For this review, use the dimensioned drawing (mm, ordinates from the lowest corner) and the shaded views. A direction names the side the tool comes from. Give positions to 0.01 mm unless a question says otherwise; leave off trailing zeros. Write each loop counter-clockwise with the first axis right and the second up, starting at its lowest first coordinate (ties: lowest second). Pieces come first, ordered by that corner, then holes. Notation, with made-up numbers: M -23,-1.5 L -4,-1.5 A8 cw -4,13.5 Z; hole C -13.5,-6.5 d1. An arc over 180 degrees is marked long. Write each question's results on one line, items separated by ' | '. Start each with the question number.
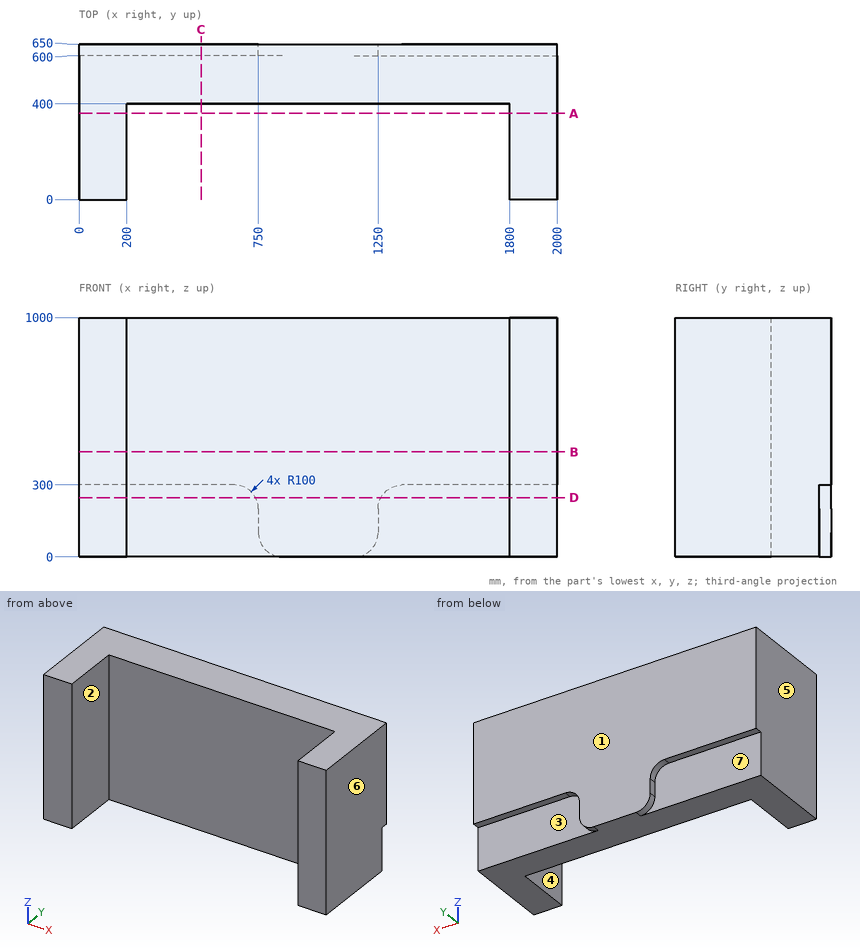
(1) Wall thickness on L1, parallel to X at y = 142, z = 559; L2, parallel to Y at x = 331, z = 341.5; L3, parallel to Y at x = 1879.5, z = 260: over which ranges is each line inside the solid? List them lowest first.
(2) Clearance check with flat-ended pins moving along their axes: P1, Ø15, axis at x = 328.5, y = 637.5, coming from the -Z side; P2, Ø25, axis at y = 615, z = 166, coming from the -X side; P3, Ø3, axis at x = 1772, z = 607.5, coming from the -Y side. State where each tip first meets the part, or that it passes through.
(3) Add section D-D (z = 247). State the section outline as (x, y) points, then the cut area to 3 significant figures.
(4) Machinability: for the marked faces 1, 2 and 3, which of the approach directions +Z, -Z, +X, -X, +Y, -Y give a long, thin tool a straight path to every point of the face, cutting with its end or side? Answer none if there is none.
(5) Draft analysis for pull direction X (two halves, no side actions). For the marked faces 4, 5, 6 and 7, state which applies: pulls with the +X half, pulls with the -X half, needs draft (parallel to the pull), parting line crosses it, or undercut.
(6) Add section B-B (z = 438). State the section outline as (x, y) points.
(7) Add section C-C (x = 510). State the section outline as (y, z) points, then the cut area to 3 significant figures.
(8) Add section A-A (y = 360). State the section outline as (x, z) points.
Calculated:
1) L1: x = 0 to 200, 1800 to 2000 | L2: y = 400 to 650 | L3: y = 0 to 600
2) P1: stops at z = 300 | P2: stops at x = 750 | P3: stops at y = 400
3) outline: M 0,0 L 200,0 L 200,400 L 1800,400 L 1800,0 L 2000,0 L 2000,600 L 1261.73,600 L 1261.73,650 L 738.27,650 L 738.27,600 L 0,600 Z | area: 586,000 mm²
4) face 1: +Z, -Z, +X, -X, +Y | face 2: +Z, -Z, -Y | face 3: -Z, +X, +Y
5) face 4: undercut | face 5: pulls with the -X half | face 6: pulls with the +X half | face 7: needs draft
6) outline: M 0,0 L 200,0 L 200,400 L 1800,400 L 1800,0 L 2000,0 L 2000,650 L 0,650 Z
7) outline: M 400,0 L 600,0 L 600,300 L 650,300 L 650,1000 L 400,1000 Z | area: 235,000 mm²
8) outline: M 0,0 L 200,0 L 200,1000 L 0,1000 Z; M 1800,0 L 2000,0 L 2000,1000 L 1800,1000 Z
